Can you work these out from the model? Positions are in its coordinate system, mm. A direction names the side the tool comes from. Give positions to 0.01 mm unless a question says otherwise; leave off trailing zeros. Loops run counter-clockwise (first coordinate to the right, second up) from the corner with the lowest first, then second, coordinate; pieces in that order, holes last. Notation, with made-up numbers: (56.25, 6.25) -> (112.25, 6.25) arc R24 ccw to (112.25, 36.25) -> close; hole circle Ø4 at (26.25, -31). An arc over 180 degrees is marked (long way). One line per question, with ' | ' between items.
from build123d import *

# Parameters (mm, degrees)
F2_SIZE       = 0.2
F3_W          = 4
F3_H          = 8
F4_DEPTH      = 7.901
F4_DEPTH_BACK = 7.901
F5_W          = 4
F5_H          = 8
F6_DEPTH      = 7.901
F6_DEPTH_BACK = 7.901


with BuildPart() as f1:
    # F0 (on Front) → F1 (revolve)
    with BuildSketch(Plane.XZ):
        Polygon((4, 0), (4, -12.1), (6.95, -12.1), (6.95, -10.1), (5.95, -10.1), (5.95, -2), (7.9, -2), (7.9, 0), align=None)
    revolve(axis=Axis((0, 0, -6.05), (0, 0, -1)))

    # F2
    f2_edges = [f1.edges().sort_by_distance(p)[0] for p in [
        (-4, 0, 0),
        (-4, 0, -12.1),
        (4, 0, -6.05),
        (-7.9, 0, -2),
        (-7.9, 0, 0),
        (7.9, 0, -1),
        (-6.95, 0, -12.1),
        (-6.95, 0, -10.1),
        (6.95, 0, -11.1),
    ]]
    chamfer(f2_edges, length=F2_SIZE)

    # F3 (on Front) → F4 (cut, two sides)
    with BuildSketch(Plane.XZ) as f4_sk:
        with Locations((0, -8.1)):
            Rectangle(F3_W, F3_H)
    extrude(amount=-F4_DEPTH, mode=Mode.SUBTRACT)
    extrude(f4_sk.sketch, amount=F4_DEPTH_BACK, mode=Mode.SUBTRACT)

    # F5 (on Right) → F6 (cut, two sides)
    with BuildSketch(Plane.YZ) as f6_sk:
        with Locations((0, -8.1)):
            Rectangle(F5_W, F5_H)
    extrude(amount=F6_DEPTH, mode=Mode.SUBTRACT)
    extrude(f6_sk.sketch, amount=-F6_DEPTH_BACK, mode=Mode.SUBTRACT)


solid = f1.part
Q1. If we mould it in two halves opening along Z, with no side actions, what happens to faces 1 (the face through (4, -5, -10.1)), 2 (the face through (0, 5, -4.1)), 3 (the face through (-4.4, -4.4, -10.1)), 4 (the face through (5, -2, -8))? For each: pulls with the +Z half, pulls with the -Z half, needs draft (parallel to the pull), parting line crosses it, or undercut.
Entries:
face 1: undercut | face 2: pulls with the -Z half | face 3: undercut | face 4: needs draft
Q2. If we section it at A-A (y = 0): Write out the boundary of the cut face in (x, z).
Entries:
outline: (-7.9, -1.8) -> (-7.7, -2) -> (-5.95, -2) -> (-5.95, -4.1) -> (-4, -4.1) -> (-4, -0.2) -> (-4.2, 0) -> (-7.7, 0) -> (-7.9, -0.2) -> close; (4, -4.1) -> (5.95, -4.1) -> (5.95, -2) -> (7.7, -2) -> (7.9, -1.8) -> (7.9, -0.2) -> (7.7, 0) -> (4.2, 0) -> (4, -0.2) -> close
Q3. If I drill on probe 1 along X at (y, z) = (0, -2.25); probe 2 along Z at (x, y) = (2.25, 7), over which ranges is the centre line in solid material (lowest first)? Write a range as from..to.
Entries:
probe 1: -5.95..-4, 4..5.95 | probe 2: -2..0
Q4. If we section it at D-D (z = -3): Write out the boundary of the cut face in (x, y).
Entries:
outline: circle Ø11.9 at (0, 0); hole circle Ø8 at (0, 0)
Q5. If we section it at C-C (z = -7.25): Write out the boundary of the cut face in (x, y), plus the area to 3 significant figures.
Entries:
outline: (-5.6, -2) arc R5.95 ccw to (-2, -5.6) -> (-2, -3.46) arc R4 cw to (-3.46, -2) -> close; (-5.6, 2) -> (-3.46, 2) arc R4 cw to (-2, 3.46) -> (-2, 5.6) arc R5.95 ccw to start; (2, -5.6) arc R5.95 ccw to (5.6, -2) -> (3.46, -2) arc R4 cw to (2, -3.46) -> close; (2, 3.46) arc R4 cw to (3.46, 2) -> (5.6, 2) arc R5.95 ccw to (2, 5.6) -> close | area: 28.8 mm²
Q6. On a 3-axis mill with a long thin cutter (end or side, diameter ignored), from which of +Z, -Z, +X, -X, +Y, -Y can I reach the whole of each face in a straight line? I mean faces 5 (the face through (-4.95, 4.88, -11.09)), 6 (the face through (-4.4, 4.4, -10.1)), 7 (the face through (-5, -2, -8)), 8 (the face through (2.7, 5.3, -5.1)), 9 (the face through (2, 5, -8)). Say none if no direction works.
Entries:
face 5: -Z, -X, +Y | face 6: -X, +Y | face 7: -Z, +X, -X | face 8: none | face 9: -Z, +Y, -Y
Q7. For pin 1 Ø2.5 at (x, y) = (5, 0) entering from -Z; pin 2 Ø6 at (x, z) = (4, -1.5) entering from -Y; pin 3 Ø1.6 at (y, z) = (5.5, -8.5) entering from +X; pin 4 Ø1.5 at (x, z) = (1, -8) entering from +Y, each with a flat end and sliding along its axis, tell me the tip position at first contact or that it passes through.
Entries:
pin 1: z = -4.1 | pin 2: y = -7.84 | pin 3: x = 3.65 | pin 4: through
